Build history of the part. All positions in model axes, mm. A direction names the side the tool comes from. Round coordinates to 2 decimals unless told otherwise and drop trailing zeros. Loops run counter-clockwise (first coordinate to the right, second up) from the corner with the lowest first, then second, coordinate; pieces in that order, holes last. Notation, with made-up numbers: M 33,36.25 L 37,36.25 A32 ccw 37,67.25 Z; hole C 18,74 d9. An arc over 180 degrees is marked long. Use one line per item in the form item = value. Start each with the question number.
```python
from build123d import *

# Parameters (mm, degrees)
SKETCH1_W           = 40
SKETCH1_H           = 20
BOSS_EXTRUDE2_DEPTH = 40
SKETCH2_W           = 2
SKETCH2_H           = 20
BOSS_EXTRUDE3_DEPTH = 7.25
SKETCH3_R           = 2
CUT_EXTRUDE1_DEPTH  = 2
FILLET3_R           = 4
SKETCH4_W           = 2
SKETCH4_H           = 20
BOSS_EXTRUDE4_DEPTH = 7.25
SKETCH5_R           = 2
CUT_EXTRUDE2_DEPTH  = 2
FILLET4_R           = 4
SKETCH6_R           = 5
BOSS_EXTRUDE5_DEPTH = 1
SKETCH7_R           = 3.5
BOSS_EXTRUDE7_DEPTH = 4
SKETCH9_R           = 5
BOSS_EXTRUDE8_DEPTH = 1
SKETCH10_R          = 3.5
BOSS_EXTRUDE9_DEPTH = 4


with BuildPart() as part:
    # Sketch1 → Boss-Extrude2 (new body)
    with BuildSketch(Plane.XY):
        Rectangle(SKETCH1_W, SKETCH1_H)
    extrude(amount=BOSS_EXTRUDE2_DEPTH)

    # Sketch2 → Boss-Extrude3 (add)
    with BuildSketch(Plane(origin=(20, 0, 0), x_dir=(0, 0, -1), z_dir=(1, 0, 0))):
        with Locations((-33, 0)):
            Rectangle(SKETCH2_W, SKETCH2_H)
    extrude(amount=BOSS_EXTRUDE3_DEPTH)

    # Sketch3 → Cut-Extrude1 (cut)
    with BuildSketch(Plane.XY.offset(34)):
        with Locations((24.75, -4.99913934)):
            Circle(SKETCH3_R)
        with Locations((24.75, 4.999429987)):
            Circle(SKETCH3_R)
    extrude(amount=-CUT_EXTRUDE1_DEPTH, mode=Mode.SUBTRACT)

    # Fillet3
    fillet3_edges = [part.edges().sort_by_distance(p)[0] for p in [
        (27.25, -10, 33),
        (27.25, 10, 33),
    ]]
    fillet(fillet3_edges, radius=FILLET3_R)

    # Sketch4 → Boss-Extrude4 (add)
    with BuildSketch(Plane.ZY.offset(20)):
        with Locations((33, 0)):
            Rectangle(SKETCH4_W, SKETCH4_H)
    extrude(amount=BOSS_EXTRUDE4_DEPTH)

    # Sketch5 → Cut-Extrude2 (cut)
    with BuildSketch(Plane.XY.offset(34)):
        with Locations((-24.75, 5)):
            Circle(SKETCH5_R)
        with Locations((-24.75, -5)):
            Circle(SKETCH5_R)
    extrude(amount=-CUT_EXTRUDE2_DEPTH, mode=Mode.SUBTRACT)

    # Fillet4
    fillet4_edges = [part.edges().sort_by_distance(p)[0] for p in [
        (-27.25, -10, 33),
        (-27.25, 10, 33),
    ]]
    fillet(fillet4_edges, radius=FILLET4_R)

    # Sketch6 → Boss-Extrude5 (add)
    with BuildSketch(Plane.XY.offset(40)):
        with Locations((-10, 0)):
            Circle(SKETCH6_R)
    extrude(amount=BOSS_EXTRUDE5_DEPTH)

    # Sketch7 → Boss-Extrude7 (add)
    with BuildSketch(Plane.XY.offset(41)):
        with Locations((-10, 0)):
            Circle(SKETCH7_R)
    extrude(amount=BOSS_EXTRUDE7_DEPTH)

    # Sketch9 → Boss-Extrude8 (add)
    with BuildSketch(Plane(origin=(0, 0, 0), x_dir=(-1, 0, 0), z_dir=(0, 0, -1))):
        with Locations((10, 0)):
            Circle(SKETCH9_R)
    extrude(amount=BOSS_EXTRUDE8_DEPTH)

    # Sketch10 → Boss-Extrude9 (add)
    with BuildSketch(Plane(origin=(0, 0, -1), x_dir=(-1, 0, 0), z_dir=(0, 0, -1))):
        with Locations((10, 0)):
            Circle(SKETCH10_R)
    extrude(amount=BOSS_EXTRUDE9_DEPTH)


solid = part.part
```
Q1. Wall check: probe 1 along Z at (x, y) = (-22, -4.5); probe 2 along X at (y, z) = (5, 35); probe 3 along Y at (x, z) = (24, 33). Give the ranges that are in metal, low to high.
Q2. Saw through at B-B (x = 24.75). Give the cut face in (y, z), and give its area (3 significant figures).
Q3. Saw through at D-D (z = -2). Give the cut face in (x, y), and give its area (3 significant figures).
Q4. Saw through at A-A (y = 0). Give the cut face in (x, z).
Q5. Pull direction Y, two halves, no side cores. Call faces 1 (the face through (-26.748, 5.088, 33.014)), 2 (the face through (-26.047, -8.859, 33.014)), 3 (the face through (-10, 0, 45)): pulls with the +Y half, pulls with the -Y half, needs draft (parallel to the pull), parting line crosses it, or undercut.
Q6. Saw through at C-C (x = -10). Give the cut face in (y, z), and give its area (3 significant figures).
Q7. Tool access for faces 4 (the face through (23, 0, 34)), 5 (the face through (-12.2, -3.3, -1)), 6 (the face through (-20, 0, 37)), 7 (the face through (20, 0, 16)), 8 (the face through (-7.8, -3.3, 41)): list every direction of +Z, -Z, +X, -X, +Y, -Y with a clear straight run to the whole face (end or side of a thin tool).
Q8. Drop flat-ended pins along their axis: P1, Ø6.5, axis at x = 24.75, y = -5, coming from the -Z side; P2, Ø6.5, axis at y = -5, z = 37, coming from the +X side; P3, Ø1.8, axis at y = -1.5, z = 36.5, coming from the -X side; P4, Ø1.5, axis at y = -7, z = 2, coming from the +X side. Give the stop position or say it passes through.
Filled in:
q1.probe_1 = 32 to 34
q1.probe_2 = -20 to 20
q1.probe_3 = -9.93 to -6.85, -3.15 to 3.15, 6.85 to 9.93
q2.outline = M -9.71,32 L -7,32 L -7,34 L -9.71,34 Z; M -3,32 L 3,32 L 3,34 L -3,34 Z; M 7,32 L 9.71,32 L 9.71,34 L 7,34 Z
q2.area = 22.8 mm²
q3.outline = C -10,0 d7
q3.area = 38.5 mm²
q4.outline = M -27.25,32 L -20,32 L -20,0 L -15,0 L -15,-1 L -13.5,-1 L -13.5,-5 L -6.5,-5 L -6.5,-1 L -5,-1 L -5,0 L 20,0 L 20,32 L 27.25,32 L 27.25,34 L 20,34 L 20,40 L -5,40 L -5,41 L -6.5,41 L -6.5,45 L -13.5,45 L -13.5,41 L -15,41 L -15,40 L -20,40 L -20,34 L -27.25,34 Z
q5.face_1 = undercut
q5.face_2 = pulls with the -Y half
q5.face_3 = needs draft
q6.outline = M -10,0 L -5,0 L -5,-1 L -3.5,-1 L -3.5,-5 L 3.5,-5 L 3.5,-1 L 5,-1 L 5,0 L 10,0 L 10,40 L 5,40 L 5,41 L 3.5,41 L 3.5,45 L -3.5,45 L -3.5,41 L -5,41 L -5,40 L -10,40 Z
q6.area = 876 mm²
q7.face_4 = +Z, +X, +Y, -Y
q7.face_5 = -Z
q7.face_6 = +Z, -X, +Y, -Y
q7.face_7 = -Z, +X, +Y, -Y
q7.face_8 = +Z
q8.P1 = 32
q8.P2 = 27.25
q8.P3 = -20
q8.P4 = 20
